Work out the finished part from the listing and answer in its coordinate system (mm). A direction names the side the tool comes from. Round coordinates to 2 decimals unless told otherwise and drop trailing zeros. Loops run counter-clockwise (first coordinate to the right, second up) from the corner with the lowest first, then second, coordinate; pieces in that order, holes last.
```python
from build123d import *

# Parameters (mm, degrees)
ESQUISSE1_R        = 17.5
BOSS_EXTRU_1_DEPTH = 10
ESQUISSE2_R        = 2
BOSS_EXTRU_2_DEPTH = 5.5
BOSS_EXTRU_3_DEPTH = 12


with BuildPart() as part:
    # Esquisse1 → Boss.-Extru.1 (new body)
    with BuildSketch(Plane.XY):
        Circle(ESQUISSE1_R)
    extrude(amount=BOSS_EXTRU_1_DEPTH)

    # Esquisse2 → Boss.-Extru.2 (add)
    with BuildSketch(Plane.XY.offset(10)):
        with Locations((8.821157095, 8.821157095)):
            Circle(ESQUISSE2_R)
        with Locations((0, 12.475)):
            Circle(ESQUISSE2_R)
        with Locations((12.475, 0)):
            Circle(ESQUISSE2_R)
        with Locations((8.821157095, -8.821157095)):
            Circle(ESQUISSE2_R)
        with Locations((0, -12.475)):
            Circle(ESQUISSE2_R)
        with Locations((-8.821157095, -8.821157095)):
            Circle(ESQUISSE2_R)
        with Locations((-12.475, 0)):
            Circle(ESQUISSE2_R)
        with Locations((-8.821157095, 8.821157095)):
            Circle(ESQUISSE2_R)
    extrude(amount=BOSS_EXTRU_2_DEPTH)

    # Esquisse3 → Boss.-Extru.3 (add)
    with BuildSketch(Plane(origin=(0, 0, 0), x_dir=(-1, 0, 0), z_dir=(0, 0, -1))):
        Polygon((11.325586205, 11.535355671), (-4.32711795, 15.575923202), (-15.652704155, 4.040567531), (-11.325586205, -11.535355671), (4.32711795, -15.575923202), (15.652704155, -4.040567531), align=None)
    extrude(amount=BOSS_EXTRU_3_DEPTH)


solid = part.part
```
1. Which of the six approach directions +Z, -Z, +X, -X, +Y, -Y give full straight-line access (tool end or side, diameter ignored) to faces 4 (the face through (10.73, 9.42, 12.71)), 5 (the face through (3.609, -13.527, -5.916)), 6 (the face through (-13.52, 3.64, -5.92)), 7 (the face through (0, 13, 15.5)), 8 (the face through (9.9, 9.9, -5.9))?
Answer key:
face 4: +Z
face 5: -Z, +X, -Y
face 6: -Z, -X, +Y
face 7: +Z, +X, -X, +Y, -Y
face 8: -Z, +X, +Y
2. Consider probe 1 along Z at (x, y) = (-0.5, 4); probe 2 along Z at (x, y) = (-10, -10.5); probe 3 along X at (y, z) = (8.5, 4.5). Determine where each line is inside the solid, lowest interval first.
Answer key:
probe 1: z = -12 to 10
probe 2: z = 0 to 10
probe 3: x = -15.3 to 15.3
3. Find section D-D (y = -2.5). Write down the section's boundary in (x, z), then the cut area to 3 significant figures.
Answer key:
outline: (-17.32, 0) - (-15.22, 0) - (-15.22, -12) - (13.84, -12) - (13.84, 0) - (17.32, 0) - (17.32, 10) - (-17.32, 10) - close
area: 695 mm2
4. Find section B-B (x = 0). Write down the section's boundary in (y, z) (3 decimals), then the cut area to 3 significant figures.
Answer key:
outline: (-17.5, 0) - (-14.459, 0) - (-14.459, -12) - (14.459, -12) - (14.459, 0) - (17.5, 0) - (17.5, 10) - (14.475, 10) - (14.475, 15.5) - (10.475, 15.5) - (10.475, 10) - (-10.475, 10) - (-10.475, 15.5) - (-14.475, 15.5) - (-14.475, 10) - (-17.5, 10) - close
area: 741 mm2
5. Find section C-C (z = 1). Write down the section's boundary in (x, y).
Answer key:
outline: circle Ø35 at (0, 0)
6. Find section A-A (y = 10). Write down the section's boundary in (x, z), then the cut area to 3 significant figures.
Answer key:
outline: (-14.36, 0) - (-11.75, 0) - (-11.75, -12) - (9.8, -12) - (9.8, 0) - (14.36, 0) - (14.36, 10) - (10.44, 10) - (10.44, 15.5) - (7.21, 15.5) - (7.21, 10) - (-7.21, 10) - (-7.21, 15.5) - (-10.44, 15.5) - (-10.44, 10) - (-14.36, 10) - close
area: 581 mm2
7. Determine the mould class of faces 1 (the face through (-10.63, -0.77, 12.71)), 2 (the face through (-3.609, 13.527, -5.916)), 3 (the face through (9, 9, 15.5)) for opening direction Y: +Y half, -Y half, draft (parallel to the pull), parting line (faces both ways), or undercut.
Answer key:
face 1: undercut
face 2: +Y half
face 3: draft
8. Given pin 1 (1 mm diameter, centred on x = 9, z = 2.5, fed in from +Y); pin 2 (3 mm diameter, centred on x = 3, z = 2, fed in from +Y); pin 3 (8 mm diameter, centred on x = 3.5, z = 11.5, fed in from -Y); pin 4 (8 mm diameter, centred on x = 9.5, z = 2.5, fed in from +Y), each flat-ended and moving along its own axis, determine where each tip first touches the part or whether it passes through.
Answer key:
pin 1: stops at y = 15.3
pin 2: stops at y = 17.44
pin 3: stops at y = -17.5
pin 4: stops at y = 16.61
